from build123d import *

# Parameters (mm, degrees)
F1_DEPTH  = 127
F2_W      = 25.4
F2_H      = 101.6
F3_DEPTH  = 25.4
F4_W      = 50.8
F4_H      = 25.4
F5_DEPTH  = 203.2
F6_R      = 3.81
F7_DEPTH  = 50.8
F8_R      = 3.81
F9_DEPTH  = 50.8
F10_W     = 38.1
F10_H     = 12.7
F11_DEPTH = 101.6
F12_R     = 3.81
F13_DEPTH = 50.8


with BuildPart() as f1:
    # F0 (on Right) → F1 (new body)
    with BuildSketch(Plane.YZ):
        with BuildLine():
            Line((-50.025108, 117.912475), (-50.025108, 29.012475))
            Line((-50.025108, 29.012475), (153.174892, 29.012475))
            ThreePointArc((153.174892, 29.012475), (57.178696, 86.271171), (-50.025108, 117.912475))
        make_face()
        with BuildLine():
            Line((153.174892, 29.012475), (-50.025108, 29.012475))
            Line((-50.025108, 29.012475), (-50.025108, -34.487525))
            Line((-50.025108, -34.487525), (-151.625108, -34.487525))
            Line((-151.625108, -34.487525), (-151.625108, -47.187525))
            ThreePointArc((-151.625108, -47.187525), (6.772136, -33.076502), (153.174892, 29.012475))
        make_face()
    extrude(amount=F1_DEPTH)

    # F2 (on face) → F3 (cut)
    with BuildSketch(Plane.XY.offset(-34.487525)):
        with Locations((76.2, -100.825108)):
            Rectangle(F2_W, F2_H)
    extrude(amount=-F3_DEPTH, mode=Mode.SUBTRACT)

    # F4 (on face) → F5 (cut)
    with BuildSketch(Plane.XZ.offset(50.025108)):
        with Locations((63.5, 79.812475)):
            Rectangle(F4_W, F4_H)
        with Locations((63.5, -9.087525)):
            Rectangle(F4_W, F4_H)
    extrude(amount=-F5_DEPTH, mode=Mode.SUBTRACT)

    # F6 (on face) → F7 (join)
    with BuildSketch(Plane.XZ.offset(151.625108)):
        with Locations((96.52, -40.837525)):
            Circle(F6_R)
        with Locations((119.38, -40.837525)):
            Circle(F6_R)
    extrude(amount=F7_DEPTH)

    # F8 (on face) → F9 (join)
    with BuildSketch(Plane.XZ.offset(151.625108)):
        with Locations((7.62, -40.837525)):
            Circle(F8_R)
        with Locations((55.88, -40.837525)):
            Circle(F8_R)
    extrude(amount=F9_DEPTH)

    # F10 (on face) → F11 (join)
    with BuildSketch(Plane.XZ.offset(50.025108)):
        with Locations((107.95, 111.562475)):
            Rectangle(F10_W, F10_H)
    extrude(amount=F11_DEPTH)

    # F12 (on face) → F13 (join)
    with BuildSketch(Plane.XZ.offset(151.625108)):
        with Locations((96.52, 111.562475)):
            Circle(F12_R)
        with Locations((119.38, 111.562475)):
            Circle(F12_R)
    extrude(amount=F13_DEPTH)


solid = f1.part
Geometry check sheet. Reference: the model listing, model coordinates, mm. A direction names the side the tool comes from. Round coordinates to 2 decimals unless told otherwise and drop trailing zeros. Loops run counter-clockwise (first coordinate to the right, second up) from the corner with the lowest first, then second, coordinate; pieces in that order, holes last. Notation, with made-up numbers: (31.25, 6) - (57.25, 6) arc R22 ccw to (57.25, 28) - close; hole circle Ø4 at (42.5, 41). An arc over 180 degrees is marked (long way). One line per question, with ' | ' between items. Start each with the question number.
1. Cross-section at A-A on x = 42. Record the cut outline in (y, z), then the cut area to 3 significant figures.
2. Draft check along Z on faces 1 (the face through (63.5, -102, -41)), 2 (the face through (62.61, 35.57, 95.06)), 3 (the face through (88.9, 6, 80)), 4 (the face through (7.12, -176.67, -37.06)). Enter one of: released by +Z, released by -Z, zero draft, split by the parting line, or undercut.
3. Cross-section at B-B on y = -86.5. Record the cut outline in (x, z), then the cut area to 3 significant figures.
4. Scan lines: line 1 (Z direction, x = 63, y = 1); line 2 (Z direction, x = 89.5, y = -151); line 3 (X direction, y = -46, z = -20). Record each from-to range of solid material in increasing order. Write a range as [from, to].
5. Cross-section at D-D on z = 87. Record the cut outline in (x, y), then the cut area to 3 significant figures.
6. Depth check by flat-ended pin: pin 1 (4 mm diameter, centred on y = -107, z = 110, fed in from -X); pin 2 (5 mm diameter, centred on x = 100, y = -89, fed in from -Z); pin 3 (3 mm diameter, centred on x = 77, y = -28, fed in from -Z). Enter the tip coordinate at first touch or a pass-through.
7. Tool access check on faces 5 (the face through (88.9, -102, -41)), 6 (the face through (31, -100, -34.488)), 7 (the face through (38.1, 6, 80)). Record the directions out of +Z, -Z, +X, -X, +Y, -Y that give a thin tool (end or side, any length) a straight path to the whole face; none if there is none.
8. Cross-section at C-C on x = 119.38. Record the cut outline in (y, z).
Taken from the geometry:
1) outline: (-151.63, -47.19) arc R511.35 ccw to (45.4, -21.79) - (-50.03, -21.79) - (-50.03, -34.49) - (-151.63, -34.49) - close; (-50.03, 3.61) - (107.33, 3.61) arc R511.35 ccw to (153.17, 29.01) arc R446.82 ccw to (95.78, 67.11) - (-50.03, 67.11) - close; (-50.03, 92.51) - (42.18, 92.51) arc R446.82 ccw to (-50.03, 117.91) - close | area: 15,200 mm²
2) face 1: zero draft | face 2: released by +Z | face 3: undercut | face 4: split by the parting line
3) outline: (0, -47.42) - (63.5, -47.42) - (63.5, -34.49) - (0, -34.49) - close; (88.9, -47.42) - (127, -47.42) - (127, -34.49) - (88.9, -34.49) - close; (88.9, 105.21) - (127, 105.21) - (127, 117.91) - (88.9, 117.91) - close | area: 1,800 mm²
4) line 1: [-34.48, -21.79], [3.61, 67.11], [92.51, 106.49] | line 2: [-47.23, -34.49], [105.21, 117.91] | line 3: [0, 38.1], [88.9, 127]
5) outline: (0, -50.03) - (38.1, -50.03) - (38.1, 55.5) - (0, 55.5) - close; (88.9, -50.03) - (127, -50.03) - (127, 55.5) - (88.9, 55.5) - close | area: 8,040 mm²
6) pin 1: x = 88.9 | pin 2: z = -47.7 | pin 3: z = -40.76
7) face 5: +Z, -Z, -Y | face 6: +Z, +X, -X, -Y | face 7: +Y, -Y
8) outline: (-202.43, -44.65) - (-151.63, -44.65) - (-151.63, -47.19) arc R511.35 ccw to (153.17, 29.01) arc R446.82 ccw to (-50.03, 117.91) - (-151.63, 117.91) - (-151.63, 115.37) - (-202.43, 115.37) - (-202.43, 107.75) - (-151.63, 107.75) - (-151.63, 105.21) - (-50.03, 105.21) - (-50.03, -34.49) - (-151.63, -34.49) - (-151.63, -37.03) - (-202.43, -37.03) - close
